Read the model definition and answer for the solid it produces. Units are mm, in the model's axes. A direction names the side the tool comes from. Round coordinates to 2 decimals unless told otherwise and drop trailing zeros. Order: outer loops, then holes, each group sorted by start corner. A loop starts at its lowest first (then second) coordinate and runs counter-clockwise, first axis right, second up. Notation, with made-up numbers: (51.25, 47.25) - (91.25, 47.25) arc R24 cw to (91.25, 72.25) - close; hole circle Ø10 at (79, 35). An arc over 180 degrees is marked (long way). One line per question, with ' | ' between items. Start each with the question number.
1) The part is cut by section B-B, the plane z = 4. Give the vertices of the cut face in (x, y), plus the area to 3 significant figures.
2) The part is cut by section A-A, the plane y = 22.5. Give the vertices of the cut face in (x, z).
3) Flat-ended cylindrical pins translate along their axes: pin 1 (5 mm diameter, centred on y = 12.5, z = -6, fed in from +X); pin 2 (2 mm diameter, centred on x = -1, y = 10.5, fed in from +Z); pin 3 (4 mm diameter, centred on y = 7, z = -2.5, fed in from +X). Find the tip coordinate at first contact, or state that the pin passes through.
4) Straight lines are drawn through the part: line 1 (X direction, y = 21.3, z = 0); line 2 (Y direction, x = 6, z = -3.25); line 3 (Y direction, x = 5, z = 9.25). For each, find the intervals that lie inside material, in ascending order. Write a range as from..to.
5) The part is cut by section C-C, the plane x = 2.25. Give the vertices of the cut face in (y, z).
6) The part is cut by section D-D, the plane y = 19.5. Give the vertices of the cut face in (x, z), plus the area to 3 significant figures.
7) For faces 1 (the flat face through (2, 20, 6)), 2 (the cylindrical face through (-6.834, 22.958, -1.517)), 3 (the flat face through (5, 6, -5)), determine the directions among +Z, -Z, +X, -X, +Y, -Y from which every point of the face is accessible in a straight line to the end or side of a thin tool.
8) The mould has two halves that part along X. Classify faces 4 (the flat face through (-5, 6, 5)), 5 (the cylindrical face through (-11.97, 1.01, 11.25)), 6 (the flat face through (15, 1, 0)), 7 (the cylindrical face through (12.03, 1.01, -11.25)): pulls with the +X half, pulls with the -X half, needs draft (parallel to the pull), parting line crosses it, or undercut.
from build123d import *

# Parameters (mm, degrees)
SKETCH_1_W          = 30
SKETCH_1_H          = 25
EXTRUDE_1_DEPTH     = 2
SKETCH_2_R          = 1.25
CUT_EXTRUDE_1_DEPTH = 20.627786426
SKETCH_3_W          = 13
SKETCH_3_H          = 13
EXTRUDE_2_DEPTH     = 4
SKETCH_4_R          = 6.5
EXTRUDE_3_DEPTH     = 8
SKETCH_5_R          = 6
EXTRUDE_4_DEPTH     = 6
SKETCH_6_R          = 7
SKETCH_6_R_2        = 5.5
EXTRUDE_5_DEPTH     = 6


with BuildPart() as part:
    # 草圖1 → 填料-伸長1 (new body)
    with BuildSketch(Plane(origin=(0, 0, 0), x_dir=(1, 0, 0), z_dir=(0, 1, 0))):
        Rectangle(SKETCH_1_W, SKETCH_1_H)
    extrude(amount=EXTRUDE_1_DEPTH)

    # 草圖2 → 除料-伸長1 (cut, through all)
    with BuildSketch(Plane(origin=(0, 2, 0), x_dir=(1, 0, 0), z_dir=(0, 1, 0))):
        with Locations((-12, 12.5)):
            Circle(SKETCH_2_R)
        with Locations((-12, -12.5)):
            Circle(SKETCH_2_R)
    cut_extrude_1 = extrude(amount=-CUT_EXTRUDE_1_DEPTH, mode=Mode.SUBTRACT)

    # 鏡射1: 除料-伸長1 across plane
    add(cut_extrude_1.mirror(Plane(origin=(0, 0, 0), x_dir=(0, 0, 1), z_dir=(1, 0, 0))), mode=Mode.SUBTRACT)

    # 草圖3 → 填料-伸長2 (add)
    with BuildSketch(Plane(origin=(0, 2, 0), x_dir=(1, 0, 0), z_dir=(0, 1, 0))):
        Rectangle(SKETCH_3_W, SKETCH_3_H)
    extrude(amount=EXTRUDE_2_DEPTH)

    # 草圖4 → 填料-伸長3 (add)
    with BuildSketch(Plane(origin=(0, 6, 0), x_dir=(1, 0, 0), z_dir=(0, 1, 0))):
        with Locations(Location((0, 0, 0), (0, 0, 270))):
            Circle(SKETCH_4_R)
    extrude(amount=EXTRUDE_3_DEPTH)

    # 草圖5 → 填料-伸長4 (add)
    with BuildSketch(Plane(origin=(0, 14, 0), x_dir=(1, 0, 0), z_dir=(0, 1, 0))):
        with Locations(Location((0, 0, 0), (0, 0, 270))):
            Circle(SKETCH_5_R)
    extrude(amount=EXTRUDE_4_DEPTH)

    # 草圖6 → 填料-伸長5 (add)
    with BuildSketch(Plane(origin=(0, 20, 0), x_dir=(1, 0, 0), z_dir=(0, 1, 0))):
        with Locations(Location((0, 0, 0), (0, 0, 270))):
            Circle(SKETCH_6_R)
        with Locations(Location((0, 0, 0), (0, 0, 270))):
            Circle(SKETCH_6_R_2, mode=Mode.SUBTRACT)
    extrude(amount=EXTRUDE_5_DEPTH)


solid = part.part
Values:
1) outline: (-15, 0) - (15, 0) - (15, 2) - (6.5, 2) - (6.5, 6) - (5.12, 6) - (5.12, 14) - (4.47, 14) - (4.47, 20) - (5.74, 20) - (5.74, 26) - (3.77, 26) - (3.77, 20) - (-3.77, 20) - (-3.77, 26) - (-5.74, 26) - (-5.74, 20) - (-4.47, 20) - (-4.47, 14) - (-5.12, 14) - (-5.12, 6) - (-6.5, 6) - (-6.5, 2) - (-15, 2) - close | area: 271 mm^2
2) outline: circle Ø14 at (0, 0); hole circle Ø11 at (0, 0)
3) pin 1: stops at x = 5.48 | pin 2: stops at z = 6.5 | pin 3: stops at x = 6.5
4) line 1: x = -7..-5.5, 5.5..7 | line 2: y = 0..6, 20..26 | line 3: y = 0..2
5) outline: (0, -12.5) - (2, -12.5) - (2, -6.5) - (6, -6.5) - (6, -6.1) - (14, -6.1) - (14, -5.56) - (20, -5.56) - (20, -6.63) - (26, -6.63) - (26, -5.02) - (20, -5.02) - (20, 5.02) - (26, 5.02) - (26, 6.63) - (20, 6.63) - (20, 5.56) - (14, 5.56) - (14, 6.1) - (6, 6.1) - (6, 6.5) - (2, 6.5) - (2, 12.5) - (0, 12.5) - close
6) outline: circle Ø12 at (0, 0) | area: 113 mm^2
7) face 1: none | face 2: +Y | face 3: -Z, +X
8) face 4: needs draft | face 5: undercut | face 6: pulls with the +X half | face 7: undercut
